Autodesk Inventor part; units mm, degrees
ref_plane "YZ Plane" through (0, 0, 0) normal (1, 0, 0) x (0, 1, 0)
ref_plane "XZ Plane" through (0, 0, 0) normal (0, 1, 0) x (-1, 0, 0)
ref_plane "XY Plane" through (0, 0, 0) normal (0, 0, 1) x (1, 0, 0)
sketch "Sketch1" plane through (0, 0, 0) normal (0, 1, 0) x (-1, 0, 0)
  circle A0 centre (9.779, 0) radius 1.9304 construction
  circle A1 centre (6.9148, 6.9148) radius 1.9304 construction
  circle A2 centre (0, 9.779) radius 1.9304 construction
  circle A3 centre (-6.9148, 6.9148) radius 1.9304 construction
  circle A4 centre (-9.779, 0) radius 1.9304 construction
  circle A5 centre (-6.9148, -6.9148) radius 1.9304 construction
  circle A6 centre (0, -9.779) radius 1.9304 construction
  circle A7 centre (6.9148, -6.9148) radius 1.9304 construction
  circle A8 centre (9.779, 0) radius 3.1242 construction
  circle A9 centre (0, 9.779) radius 3.1242 construction
  circle A10 centre (-9.779, 0) radius 3.1242 construction
  circle A11 centre (0, -9.779) radius 3.1242 construction
  circle A12 centre (0, 0) radius 13.97
  circle A13 centre (6.9148, -6.9148) radius 1.9304
  circle A14 centre (6.9148, 6.9148) radius 1.9304
  circle A15 centre (-6.9148, 6.9148) radius 1.9304
  circle A16 centre (-6.9148, -6.9148) radius 1.9304
  dimension "d0" = 3.8608
  dimension "d1" = 9.779
  dimension "d4" = 360
  dimension "d6" = 6.2484
  dimension "d9" = 360
  dimension "d11" = 27.94
  dimension "d12" = 3.8608
  dimension "d13" = 3.8608
  dimension "d14" = 3.8608
  dimension "d15" = 3.8608
extrude "Extrusion1" add sketch "Sketch1" along normal blind 8.1788
hole "Hole1" at (0, 0, 9.779) at (9.779, 0, 0) at (0, 0, -9.779) at (-9.779, 0, 0) direction (0, 1, 0) diameter 3.8608 end through all counterbore diameter 6.2484 counterbore depth 4.953
properties part number "Collector rotation xrail to turntable adapter"
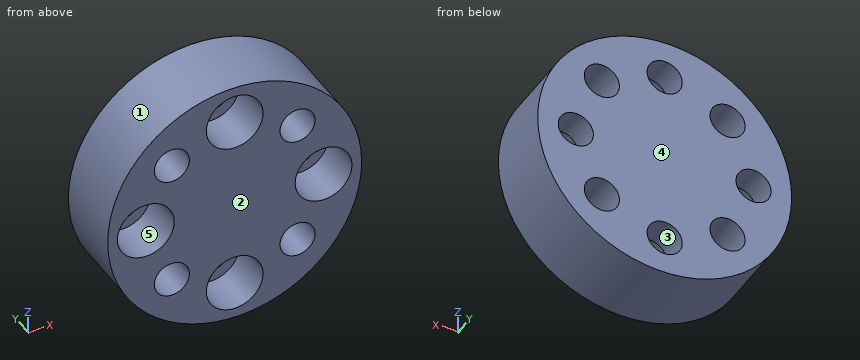
Read the model definition and answer for the solid it produces. Units are mm, in the model's axes. Face numbers are marked on the shaded views. A direction names the side the tool comes from. Coordinates: 2 decimals unless noted, no trailing zeros. Write each loop counter-clockwise with the first axis right and the second up, starting at its lowest first coordinate (ties: lowest second). Pieces come first, ordered by that corner, then holes. Notation, with made-up numbers: (-38.5, 82) -> (-17.5, 82) arc R28 ccw to (-17.5, 117) -> close; hole circle Ø3 at (87.5, -26.5). An arc over 180 degrees is marked (long way). Return JSON: item names as keys, results as strings.
1. A cutting plane is placed at C-C (y = 6.5). Give the number of separate pieces and of enclosed holes in the cut face, and give its area (3 significant figures).
Found:
{"separate pieces": "1", "enclosed holes": "8", "area": "519 mm2"}
2. A cutting plane is placed at D-D (z = 5.75). Determine the outline of the cut face in (x, y).
Found:
{"outline": "(-12.73, 0) -> (-8.45, 0) -> (-8.45, 8.18) -> (-12.73, 8.18) -> close; (-5.38, 0) -> (5.38, 0) -> (5.38, 8.18) -> (-5.38, 8.18) -> close; (8.45, 0) -> (12.73, 0) -> (12.73, 8.18) -> (8.45, 8.18) -> close"}
3. Determine the mould class of the marked faces 1, 2 and 3 for opening direction X: pulls with the +X half, pulls with the -X half, needs draft (parallel to the pull), parting line crosses it, or undercut.
Found:
{"face 1": "parting line crosses it", "face 2": "needs draft", "face 3": "undercut"}
4. A cutting plane is placed at B-B (z = 0). Determine the outline of the cut face in (x, y), and give its area (3 significant figures).
Found:
{"outline": "(-13.97, 0) -> (-12.9, 0) -> (-12.9, 4.95) -> (-11.71, 4.95) -> (-11.71, 8.18) -> (-13.97, 8.18) -> close; (-7.85, 4.95) -> (-6.65, 4.95) -> (-6.65, 0) -> (6.65, 0) -> (6.65, 4.95) -> (7.85, 4.95) -> (7.85, 8.18) -> (-7.85, 8.18) -> close; (11.71, 4.95) -> (12.9, 4.95) -> (12.9, 0) -> (13.97, 0) -> (13.97, 8.18) -> (11.71, 8.18) -> close", "area": "142 mm2"}
5. A cutting plane is placed at A-A (x = 0). Determine the outline of the cut face in (y, z), and give its area (3 significant figures).
Found:
{"outline": "(0, -13.97) -> (8.18, -13.97) -> (8.18, -11.71) -> (4.95, -11.71) -> (4.95, -12.9) -> (0, -12.9) -> close; (0, -6.65) -> (4.95, -6.65) -> (4.95, -7.85) -> (8.18, -7.85) -> (8.18, 7.85) -> (4.95, 7.85) -> (4.95, 6.65) -> (0, 6.65) -> close; (0, 12.9) -> (4.95, 12.9) -> (4.95, 11.71) -> (8.18, 11.71) -> (8.18, 13.97) -> (0, 13.97) -> close", "area": "142 mm2"}
6. Find the intervals of material crossed by line 1 along Z through (x, y) = (0, 7.2); line 2 along Z through (x, y) = (6, 4.5); line 3 along Z through (x, y) = (-8.5, 3), in increasing order. Write a range as from..to.
Found:
{"line 1": "-13.97..-11.71, -7.85..7.85, 11.71..13.97", "line 2": "-12.62..-8.61, -5.21..5.21, 8.61..12.62", "line 3": "-11.09..-8.02, -5.81..-2.85, 2.85..5.81, 8.02..11.09"}
7. A tool of negligible diameter and unlimited length cuts with its end or side. For the marked faces 4 and 5, from which of +Z, -Z, +X, -X, +Y, -Y can it reach the whole face along a straight path? Write none if from no direction.
Found:
{"face 4": "+Z, -Z, +X, -X, +Y", "face 5": "-Y"}
8. Each of these flat-tipped pins is pushed along its axis until it touches: P1, Ø6, axis at x = 9.779, z = 0, coming from the -Y side; P2, Ø12, axis at x = 8.5, z = 2, coming from the -Y side; P3, Ø1, axis at x = 4.5, y = 3.5, coming from the +Z side. Where does it stop, or does it pass through?
Found:
{"P1": "y = 4.95", "P2": "y = 0", "P3": "z = 13.39"}
